Build history of the part. All positions in model axes, mm. A direction names the side the tool comes from. Round coordinates to 2 decimals unless told otherwise and drop trailing zeros. Write each loop counter-clockwise with the first axis right and the second up, starting at its lowest first coordinate (ties: lowest second). Pieces come first, ordered by that corner, then holes.
from build123d import *

# Parameters (mm, degrees)
SKETCH_1_R          = 2.95
EXTRUDE_1_DEPTH     = 2.7
SKETCH_2_R          = 1.5
EXTRUDE_2_DEPTH     = 20
SKETCH_3_R          = 1.25
EXTRUDE_3_DEPTH     = 5
CUT_EXTRUDE_1_DEPTH = 2
FILLET_1_R          = 0.2


with BuildPart() as part:
    # 草图1 → 凸台-拉伸1 (new body)
    with BuildSketch(Plane(origin=(0, 0, 0), x_dir=(1, 0, 0), z_dir=(0, 1, 0))):
        Circle(SKETCH_1_R)
    extrude(amount=EXTRUDE_1_DEPTH)

    # 草图2 → 凸台-拉伸2 (add)
    with BuildSketch(Plane(origin=(0, 2.7, 0), x_dir=(1, 0, 0), z_dir=(0, 1, 0))):
        Circle(SKETCH_2_R)
    extrude(amount=EXTRUDE_2_DEPTH)

    # 草图3 → 凸台-拉伸3 (add)
    with BuildSketch(Plane(origin=(0, 22.7, 0), x_dir=(1, 0, 0), z_dir=(0, 1, 0))):
        Circle(SKETCH_3_R)
    extrude(amount=EXTRUDE_3_DEPTH)

    # 草图4 → 切除-拉伸1 (cut)
    with BuildSketch(Plane.XZ):
        Polygon((2.247285488, -0.53201623), (1.584382314, 1.680198207), (-0.662903174, 2.212214437), (-2.247285488, 0.53201623), (-1.584382314, -1.680198207), (0.662903174, -2.212214437), align=None)
    extrude(amount=-CUT_EXTRUDE_1_DEPTH, mode=Mode.SUBTRACT)

    # 圆角1
    fillet_1_edges = [part.edges().sort_by_distance(p)[0] for p in [
        (-1.25, 27.7, 0),
        (-2.95, 0, 0),
        (-2.95, 2.7, 0),
    ]]
    fillet(fillet_1_edges, radius=FILLET_1_R)


solid = part.part
1) Wall check: L1, parallel to Y at x = 1.4, z = -1.7; L2, parallel to Y at x = -1.4, z = -0.3; L3, parallel to Z at x = 0.1, y = 12.5. Give the ranges that are in metal, low to high.
Results:
L1: y = 0 to 2.7
L2: y = 2 to 22.7
L3: z = -1.5 to 1.5
2) Pin check, flat tips, straight feed: pin 1 Ø3 at (y, z) = (18.5, 1) entering from +X; pin 2 Ø2 at (x, z) = (0, -0.5) entering from -Y; pin 3 Ø3 at (x, y) = (0.5, 19) entering from +Z. Stop position of each tip, or through.
Results:
pin 1: stops at x = 1.5
pin 2: stops at y = 2
pin 3: stops at z = 1.5
3) Slice it at B-B (x = 0). Write the cut outline in (y, z).
Results:
outline: (0, -2.75) arc R0.2 ccw to (0.2, -2.95) - (2.5, -2.95) arc R0.2 ccw to (2.7, -2.75) - (2.7, -1.5) - (22.7, -1.5) - (22.7, -1.25) - (27.5, -1.25) arc R0.2 ccw to (27.7, -1.05) - (27.7, 1.05) arc R0.2 ccw to (27.5, 1.25) - (22.7, 1.25) - (22.7, 1.5) - (2.7, 1.5) - (2.7, 2.75) arc R0.2 ccw to (2.5, 2.95) - (0.2, 2.95) arc R0.2 ccw to (0, 2.75) - (0, 2.06) - (2, 2.06) - (2, -2.06) - (0, -2.06) - close
4) Mould opens along X. For faces 4 (the flat face through (0.48, 0.99, 1.94)), 5 (the flat face through (0, 27.7, 0)), 6 (the cylindrical face through (-2.947, 1.334, -0.13)), 7 (the flat face through (1.444, 0.986, -1.384)) say: released by +X, released by -X, zero draft, split by the parting line, or undercut.
Results:
face 4: undercut
face 5: zero draft
face 6: split by the parting line
face 7: undercut
5) Slice it at C-C (y = 26). Write the cut outline in (x, z), plus the area to 3 significant figures.
Results:
outline: circle Ø2.5 at (0, 0)
area: 4.91 mm2
6) Which spindle directions (+Z, -Z, +X, -X, +Y, -Y) get a long thin tool onto all of the face, cutting with end or side? Do faces 1 (the flat face through (0, 2, 0)), 2 (the flat face through (-2, 0, -1)), 3 (the cylindrical face through (-0.27, 25.07, 1.22)). Say none if no direction does.
Results:
face 1: -Y
face 2: +Z, -Z, +X, -X, -Y
face 3: +Y
7) Slice it at D-D (y = 3). Write the cut outline in (x, z), plus the area to 3 significant figures.
Results:
outline: circle Ø3 at (0, 0)
area: 7.07 mm2
8) Slice it at A-A (z = 0). Write the cut outline in (x, y).
Results:
outline: (-2.95, 0.2) arc R0.2 ccw to (-2.75, 0) - (-2.09, 0) - (-2.09, 2) - (2.09, 2) - (2.09, 0) - (2.75, 0) arc R0.2 ccw to (2.95, 0.2) - (2.95, 2.5) arc R0.2 ccw to (2.75, 2.7) - (1.5, 2.7) - (1.5, 22.7) - (1.25, 22.7) - (1.25, 27.5) arc R0.2 ccw to (1.05, 27.7) - (-1.05, 27.7) arc R0.2 ccw to (-1.25, 27.5) - (-1.25, 22.7) - (-1.5, 22.7) - (-1.5, 2.7) - (-2.75, 2.7) arc R0.2 ccw to (-2.95, 2.5) - close
